Source: CAD feature listing. Evaluate the final solid. Frame: model axes, mm. Face numbers are marked on the shaded views. A direction names the side the tool comes from. Give positions to 0.01 mm unless a question says otherwise; leave off trailing zeros. Write each loop counter-clockwise with the first axis right and the second up, starting at its lowest first coordinate (ties: lowest second). Pieces come first, ordered by that corner, then holes. Notation, with made-up numbers: M 71.25,84 L 79.25,84 A22 cw 79.25,112 Z; hole C -32,80 d11. An arc over 180 degrees is marked long. Use CSV: the item, a comma, the result in double quotes. Start each with the question number.
from build123d import *

# Parameters (mm, degrees)
F0_W     = 25
F0_H     = 30
F1_DEPTH = 6.5
F2_R     = 1.5
F3_DEPTH = 6.501
F4_W     = 25
F4_H     = 6.1
F5_DEPTH = 0.7
F6_SIZE  = 10
F7_R     = 10


with BuildPart() as f1:
    # F0 (on Top) → F1 (new body)
    with BuildSketch(Plane.XY):
        Rectangle(F0_W, F0_H)
    extrude(amount=F1_DEPTH)

    # F2 (on face) → F3 (cut, through all)
    with BuildSketch(Plane.XY.offset(6.5)):
        with Locations((-2, -12)):
            Circle(F2_R)
        with Locations((4.5, -1.5)):
            Circle(F2_R)
        with Locations((4.5, 8.5)):
            Circle(F2_R)
    extrude(amount=-F3_DEPTH, mode=Mode.SUBTRACT)

    # F4 (on face) → F5 (cut)
    with BuildSketch(Plane.XY.offset(6.5)):
        with Locations((0, 3.051)):
            Rectangle(F4_W, F4_H)
    extrude(amount=-F5_DEPTH, mode=Mode.SUBTRACT)

    # F6
    f6_edges = [f1.edges().sort_by_distance(p)[0] for p in [
        (-12.5, 15, 3.25),
    ]]
    chamfer(f6_edges, length=F6_SIZE)

    # F7
    f7_edges = [f1.edges().sort_by_distance(p)[0] for p in [
        (-2.5, 15, 3.25),
        (-12.5, 5, 2.9),
        (12.5, 15, 3.25),
    ]]
    fillet(f7_edges, radius=F7_R)


solid = f1.part
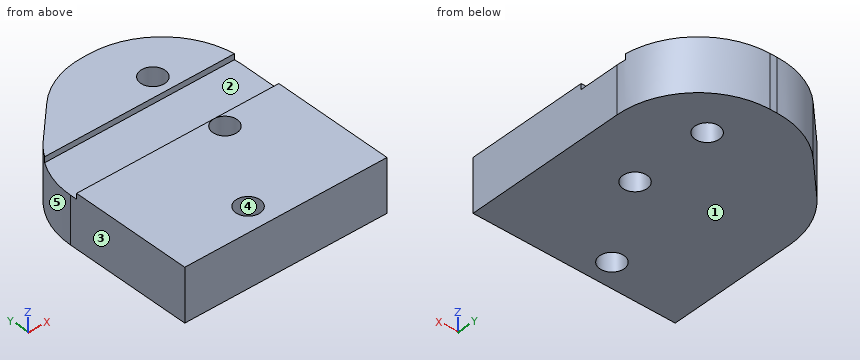
Item 1: Section B-B (z = 1). Return the cut outline in (x, y).
Item 2: Section C-C (x = 4.5). State how many separate pieces and enclosed holes the cut face has, plus the area to 3 significant figures.
Item 3: Set-up query: the marked faces 1 and 2. Return all of +Z, -Z, +X, -X, +Y, -Y with unobstructed straight access to the full face (end or side cutting, diameter ignored); none if empty.
Item 4: Pull-direction query (Y, two-part tool) for the marked faces 3, 4 and 5; classes: released by +Y, released by -Y, zero draft, split by the parting line, or undercut.
Item 5: Material intervals for probe 1 along Y at (x, z) = (4.5, 5.25); probe 2 along Y at (x, z) = (3.75, 3.75); probe 3 along Z at (x, y) = (-10.25, 5.75), sorted ascending.
Item 6: Section D-D (x = 2). Return the cut outline in (y, z), plus the area to 3 significant figures.
Item 7: Section A-A (y = -1.5). Return the cut outline in (x, z).
Output values:
1,outline,"M -12.5,-15 L 12.5,-15 L 12.5,5 A10 ccw 2.5,15 L 1.64,15 A10 ccw -5.43,12.07 L -9.57,7.93 A10 ccw -12.5,0.86 Z; hole C -2,-12 d3; hole C 4.5,-1.5 d3; hole C 4.5,8.5 d3"
2,separate pieces,"3"
2,enclosed holes,"0"
2,area,"150 mm2"
3,face 1,"-Z, +X, -X, +Y, -Y"
3,face 2,"+Z, +X, -X"
4,face 3,"zero draft"
4,face 4,"undercut"
4,face 5,"released by +Y"
5,probe 1,"y = -15 to -3, 0 to 7, 10 to 14.8"
5,probe 2,"y = -15 to -2.8, -0.2 to 7.2, 9.8 to 14.92"
5,probe 3,"z = 0 to 5.8"
6,outline,"M -15,0 L 15,0 L 15,6.5 L 6.1,6.5 L 6.1,5.8 L 0,5.8 L 0,6.5 L -15,6.5 Z"
6,area,"191 mm2"
7,outline,"M -12.5,0 L 3,0 L 3,6.5 L -12.5,6.5 Z; M 6,0 L 12.5,0 L 12.5,6.5 L 6,6.5 Z"
